```python
from build123d import *

# Parameters (mm, degrees)
SKETCH1_W           = 110
SKETCH1_H           = 5
BOSS_EXTRUDE1_DEPTH = 200
SKETCH2_W           = 25
SKETCH2_H           = 5
BOSS_EXTRUDE2_DEPTH = 5
SKETCH4_W           = 30.2
SKETCH4_H           = 5.2
CUT_EXTRUDE1_DEPTH  = 5
SKETCH5_W           = 4.2
SKETCH5_H           = 5.2
SKETCH5_W_2         = 10
SKETCH5_H_2         = 10
SKETCH5_H_3         = 5
CUT_EXTRUDE2_DEPTH  = 10
SKETCH6_W           = 10
SKETCH6_H           = 5
CUT_EXTRUDE3_DEPTH  = 5
SKETCH7_W           = 10
SKETCH7_H           = 9
CUT_EXTRUDE4_DEPTH  = 10


with BuildPart() as part:
    # Sketch1 → Boss-Extrude1 (new body)
    with BuildSketch(Plane.XY):
        with Locations((-55, 2.5)):
            Rectangle(SKETCH1_W, SKETCH1_H)
    extrude(amount=BOSS_EXTRUDE1_DEPTH)

    # Sketch2 → Boss-Extrude2 (add)
    with BuildSketch(Plane(origin=(0, 5, 0), x_dir=(1, 0, 0), z_dir=(0, 1, 0))):
        with Locations((-82.5, 2.5)):
            Rectangle(SKETCH2_W, SKETCH2_H)
        with Locations((-27.5, 2.5)):
            Rectangle(SKETCH2_W, SKETCH2_H)
        with Locations((-27.5, -202.5)):
            Rectangle(SKETCH2_W, SKETCH2_H)
        with Locations((-82.5, -202.5)):
            Rectangle(SKETCH2_W, SKETCH2_H)
    extrude(amount=-BOSS_EXTRUDE2_DEPTH)

    # Sketch4 → Cut-Extrude1 (cut)
    with BuildSketch(Plane(origin=(0, 5, 0), x_dir=(1, 0, 0), z_dir=(0, 1, 0))):
        with Locations((-55, -27.6)):
            Rectangle(SKETCH4_W, SKETCH4_H)
        with Locations((-55, -42.6)):
            Rectangle(SKETCH4_W, SKETCH4_H)
        with Locations((-55, -57.6)):
            Rectangle(SKETCH4_W, SKETCH4_H)
    extrude(amount=-CUT_EXTRUDE1_DEPTH, mode=Mode.SUBTRACT)

    # Sketch5 → Cut-Extrude2 (cut)
    with BuildSketch(Plane(origin=(0, 5, 0), x_dir=(1, 0, 0), z_dir=(0, 1, 0))):
        with Locations((-55, -2.6)):
            Rectangle(SKETCH5_W, SKETCH5_H)
        with Locations((-55, -10.2)):
            Rectangle(SKETCH5_W_2, SKETCH5_H_2)
        with Locations((-55, -197.5)):
            Rectangle(SKETCH5_W, SKETCH5_H_3)
        with Locations((-55, -190)):
            Rectangle(SKETCH5_W_2, SKETCH5_H_2)
    extrude(amount=-CUT_EXTRUDE2_DEPTH, mode=Mode.SUBTRACT)

    # Sketch6 → Cut-Extrude3 (cut)
    with BuildSketch(Plane(origin=(0, 5, 0), x_dir=(1, 0, 0), z_dir=(0, 1, 0))):
        with Locations((-105, -22.5)):
            Rectangle(SKETCH6_W, SKETCH6_H)
        with Locations((-5, -22.5)):
            Rectangle(SKETCH6_W, SKETCH6_H)
    extrude(amount=-CUT_EXTRUDE3_DEPTH, mode=Mode.SUBTRACT)

    # Sketch7 → Cut-Extrude4 (cut)
    with BuildSketch(Plane.XZ):
        with Locations((-5, 15.5)):
            Rectangle(SKETCH7_W, SKETCH7_H)
        with Locations((-105, 15.5)):
            Rectangle(SKETCH7_W, SKETCH7_H)
    extrude(amount=-CUT_EXTRUDE4_DEPTH, mode=Mode.SUBTRACT)


solid = part.part
```
Check sheet for the modelled part. Datum: model origin and axes. Units: mm. A direction names the side the tool comes from. Round coordinates to 2 decimals unless told otherwise and drop trailing zeros. Order: outer loops, then holes, each group sorted by start corner. A loop starts at its lowest first (then second) coordinate and runs counter-clockwise, first axis right, second up. Notation, with made-up numbers: M 16,50.25 L 30,50.25 A22 cw 30,79.25 Z; hole C 6.25,26 d5. An arc over 180 degrees is marked long. Answer in a Markdown table with one row per item.
(1) Section check A-A on x = -55. Record the boundary of the cut face in (y, z), plus the area to 3 significant figures.
Findings:
| item | result |
|---|---|
| outline | M 0,15.2 L 5,15.2 L 5,25 L 0,25 Z; M 0,30.2 L 5,30.2 L 5,40 L 0,40 Z; M 0,45.2 L 5,45.2 L 5,55 L 0,55 Z; M 0,60.2 L 5,60.2 L 5,185 L 0,185 Z |
| area | 771 mm^2 |
(2) Gauge pin test, flat ends, axial feed: pin 1 (1.5 mm diameter, centred on y = 1.5, z = 201.5, fed in from -X); pin 2 (1.5 mm diameter, centred on y = 1.5, z = 203.5, fed in from +X); pin 3 (3 mm diameter, centred on x = -58.5, y = 1.5, fed in from -Z). Record the tip position at first contact, or that the pin passes through.
Findings:
| item | result |
|---|---|
| pin 1 | stops at x = -95 |
| pin 2 | stops at x = -15 |
| pin 3 | stops at z = 0 |
(3) Set-up check for faces 1 (the flat face through (-39.9, 3, 28)), 2 (the flat face through (-8, 3, 200)), 3 (the flat face through (-64, 3, 200)), 4 (the flat face through (-52.9, 3, 3)): record each of +Z, -Z, +X, -X, +Y, -Y from which the full face is reachable in a straight line by a thin tool's end or side.
Findings:
| item | result |
|---|---|
| face 1 | +Y, -Y |
| face 2 | +Z, +X, +Y, -Y |
| face 3 | +Z, +Y, -Y |
| face 4 | -Z, +Y, -Y |
(4) Material ranges on line 1 along Z through (x, y) = (-41.5, 3.9); line 2 along X through (y, z) = (2.1, 191); line 3 along Z through (x, y) = (-52.5, 0.4), recorded low to high. Write a range as from..to.
Findings:
| item | result |
|---|---|
| line 1 | z = 0..25, 30.2..40, 45.2..55, 60.2..200 |
| line 2 | x = -110..-60, -50..0 |
| line 3 | z = 0..5.2, 15.2..25, 30.2..40, 45.2..55, 60.2..185, 195..200 |
(5) Section check B-B on y = 1.2. Give the number of separate pieces and of enclosed holes in the cut face, plus the area to 3 significant figures.
Findings:
| item | result |
|---|---|
| separate pieces | 1 |
| enclosed holes | 3 |
| area | 21,500 mm^2 |
(6) Draft check along X on faces 5 (the flat face through (-103, 3, 200)), 6 (the flat face through (-39.9, 3, 58)), 7 (the flat face through (-95, 3, -2)), 8 (the flat face through (-70.1, 3, 28)). Enter one of: +X half, -X half, draft (parallel to the pull), parting line (faces both ways), or undercut.
Findings:
| item | result |
|---|---|
| face 5 | draft |
| face 6 | undercut |
| face 7 | -X half |
| face 8 | undercut |
